Geometry check sheet. Reference: drawing and pictorial views, mm from the part's lowest x, y, z. Give positions to 0.01 mm unless a question says otherwise; leave off trailing zeros. Order: outer loops, then holes, each group sorted by start corner. A loop starts at its lowest first (then second) coordinate and runs counter-clockwise, first axis right, second up.
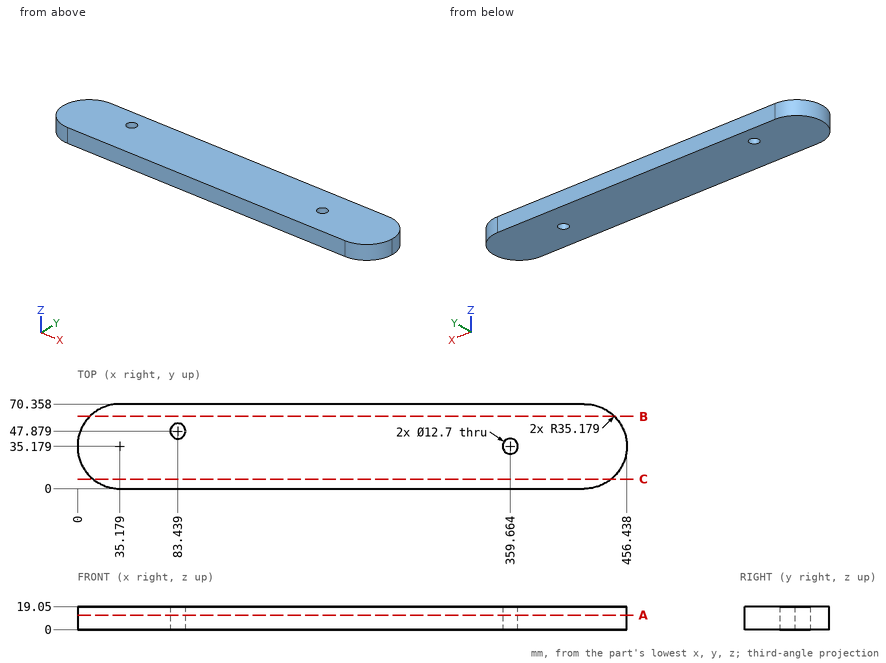
(1) Sectioned sample at C-C (y = 8). Enter the section's corners in (x, z).
(2) Sectioned sample at A-A (z = 12). Count the separate pieces of the cut face and the enclosed holes in it, plus the area to 3 significant figures.
(3) Thickness scan on L1, parallel to X at y = 34.5, z = 16; L2, parallel to Y at x = 80.5, z = 16.25; L3, parallel to X at y = 47.5, z = 7.5. Record the ranges inside material, lowest first.
(4) Go/stop test with flat-tipped pins: P1, Ø6, axis at y = 42, z = 5.5, coming from the +X side; P2, Ø4, axis at y = 19, z = 11, coming from the -X side; P3, Ø6, axis at y = 58, z = 5, coming from the -X side. Record where each tip stops, or that it passes through.
(5) Sectioned sample at B-B (y = 60). Enter the section's corners in (x, z), plus the area to 3 significant figures.
Values follow:
1. outline: (12.84, 0) - (443.59, 0) - (443.59, 19.05) - (12.84, 19.05) - close
2. separate pieces: 1
2. enclosed holes: 2
2. area: 30,800 mm2
3. L1: x = 0.01 to 353.35, 365.98 to 456.43
3. L2: y = 0 to 42.25, 53.51 to 70.36
3. L3: x = 2.23 to 77.1, 89.78 to 454.21
4. P1: stops at x = 456.23
4. P2: stops at x = 2.98
4. P3: stops at x = 6.12
5. outline: (10.25, 0) - (446.19, 0) - (446.19, 19.05) - (10.25, 19.05) - close
5. area: 8,300 mm2
